```python
from build123d import *

# Parameters (mm, degrees)
F0_W     = 5
F0_H     = 12
F0_R     = 1
F1_DEPTH = 1
F0_W_2   = 3
F2_DEPTH = 25
F3_R     = 4
F3_R_2   = 1
F4_DEPTH = 3
F5_R     = 5.99999


# Not quite as in the source:
# - a fillet or chamfer is up to 0.001 mm smaller than in the source, because OpenCascade refuses the exact size


with BuildPart() as f1:
    # F0 (on Top) → F1 (new body)
    with BuildSketch(Plane.XY):
        with Locations((-14.9452780058, -4.4979301263)):
            Rectangle(F0_W, F0_H)
        with Locations((-14.9452780058, -4.4979301263)):
            Circle(F0_R, mode=Mode.SUBTRACT)
    extrude(amount=F1_DEPTH)

    # F0 (on Top) → F2 (join)
    with BuildSketch(Plane.XY):
        with Locations((-10.9452780058, -4.4979301263)):
            Rectangle(F0_W_2, F0_H)
    extrude(amount=F2_DEPTH)

    # F3 (on face) → F4 (cut)
    with BuildSketch(Plane.YZ.offset(-9.4452780058)):
        with Locations((-4.4979301263, 19)):
            Circle(F3_R)
        with Locations((-4.4979301263, 12)):
            Circle(F3_R_2)
        with Locations((-4.4979301263, 6)):
            Circle(F3_R_2)
    extrude(amount=-F4_DEPTH, mode=Mode.SUBTRACT)

    # F5 (radius 6 in the source; OpenCascade refuses exactly that, so slightly less here)
    f5_edges = [f1.edges().sort_by_distance(p)[0] for p in [
        (-10.945278, 1.50207, 25),
        (-10.945278, -10.49793, 25),
    ]]
    fillet(f5_edges, radius=F5_R)


solid = f1.part
```
Source: CAD feature listing. Evaluate the final solid. Frame: model axes, mm. A direction names the side the tool comes from. Coordinates: 2 decimals unless noted, no trailing zeros. Loops run counter-clockwise (first coordinate to the right, second up) from the corner with the lowest first, then second, coordinate; pieces in that order, holes last. Notation, with made-up numbers: M 4,1 L 58,1 A21 cw 58,27 Z; hole C 87,42 d3. An arc over 180 degrees is marked long. Put each result on its own line as item: value. Start each with the question number.
1) Cut plane B-B on x = -11. Give the number of separate pieces and of enclosed holes in the cut face, then the cut area to 3 significant figures.
2) Cut plane A-A on z = 6. Return the cut outline in (x, y), then the cut area to 3 significant figures.
3) Pull-direction query (X, two-part tool) for faces 3 (the face through (-13.99, -4.2, 0.49)), 4 (the face through (-17.445, -4.6, 0.5)), 5 (the face through (-10.924, -0.209, 23.196)), 6 (the face through (-9.445, -5, 10)); classes: pulls with the +X half, pulls with the -X half, needs draft (parallel to the pull), parting line crosses it, or undercut.
4) Reachability of faces 1 (the face through (-10.924, -8.787, 23.196)), 2 (the face through (-12.445, -5, 10)) from +Z, -Z, +X, -X, +Y, -Y: full face, straight path, thin tool, end or side. Return the list, or none.
5) Contact query for flat-ended pins moving along their axis: pin 1 Ø3 at (x, y) = (-14.95, -4.5) entering from +Z; pin 2 Ø7 at (y, z) = (-4.5, 19) entering from -X; pin 3 Ø2.5 at (y, z) = (-4.5, 6) entering from -X. Output: stop coordinate, or through.
6) Cut plane C-C on y = -7. Return the cut outline in (x, z).
7) Cut plane D-D on z = 11.25. Return the cut outline in (x, y).
8) Ray query, L1, parallel to X at y = -5, z = 3.75; L2, parallel to Z at x = -15.5, y = -0.25; L3, parallel to Z at x = -11, y = -8. Return the intervals inside material, ascending. Write a range as from..to.
The answers:
1. separate pieces: 1
1. enclosed holes: 3
1. area: 228 mm²
2. outline: M -12.45,-10.5 L -9.45,-10.5 L -9.45,-5.5 L -12.45,-5.5 Z; M -12.45,-3.5 L -9.45,-3.5 L -9.45,1.5 L -12.45,1.5 Z
2. area: 30.0 mm²
3. face 3: undercut
3. face 4: pulls with the -X half
3. face 5: needs draft
3. face 6: pulls with the +X half
4. face 1: +Z, +X, -X, -Y
4. face 2: +Z, -X, +Y, -Y
5. pin 1: stops at z = 1
5. pin 2: passes through
5. pin 3: stops at x = -12.45
6. outline: M -17.45,0 L -9.45,0 L -9.45,15.88 L -12.45,15.88 L -12.45,1 L -17.45,1 Z; M -12.45,22.12 L -9.45,22.12 L -9.45,24.45 L -12.45,24.45 Z
7. outline: M -12.45,-10.5 L -9.45,-10.5 L -9.45,-5.16 L -12.45,-5.16 Z; M -12.45,-3.84 L -9.45,-3.84 L -9.45,1.5 L -12.45,1.5 Z
8. L1: x = -12.45..-9.45
8. L2: z = 0..1
8. L3: z = 0..17.07, 20.93..23.87
